from build123d import *

# Parameters (mm, degrees)
SKETCH1_R           = 1
BOSS_EXTRUDE1_DEPTH = 3
FILLET2_R           = 10


with BuildPart() as part:
    # Sketch1 → Boss-Extrude1 (new body)
    with BuildSketch(Plane.XY):
        with BuildLine():
            Line((0, 0), (5, 0))
            Line((5, 0), (5, -3))
            Line((5, -3), (20, -3))
            Line((20, -3), (20, 0))
            Line((20, 0), (25, 0))
            Line((25, 0), (25, 30))
            ThreePointArc((25, 30), (21.635660943, 33.364339057), (18.271321885, 30))
            Line((18.271321885, 30), (18.271321885, 25.388028695))
            Line((18.271321885, 25.388028695), (17.277972917, 24.007768839))
            ThreePointArc((17.277972917, 24.007768839), (2.760122096, 20.009620418), (3.579412381, 4.97359878))
            Line((3.579412381, 4.97359878), (0, 0))
        make_face()
        with Locations((12.5, 13)):
            Circle(SKETCH1_R, mode=Mode.SUBTRACT)
        with Locations((21.635660943, 30)):
            Circle(SKETCH1_R, mode=Mode.SUBTRACT)
    extrude(amount=BOSS_EXTRUDE1_DEPTH)

    # Fillet2
    # the kernel refuses this fillet: 10 mm, written as the material it adds along each edge
    with BuildSketch(Plane(origin=(3.579412381, 4.97359878, 0), x_dir=(-0.5841350348464551, -0.8116564920364591, 0), z_dir=(0, 0, 1))) as fillet2_piece_1_section:
        with BuildLine():
            CenterArc((6.344003322, -9.997660671), FILLET2_R, 91.239343662, 53.979959966)
            Line((-1.869411105, -4.293291867), (-2.033679393, -4.179204491))
            ThreePointArc((-2.033679393, -4.179204491), (-0.906628796, -2.158871285), (-0.19542514, 0.042532512))
            Line((-0.19542514, 0.042532512), (0, 0.2))
            ThreePointArc((0, 0.2), (3.063856958, 0.2), (6.123388127, 0.199953213))
            Line((6.123388127, 0.199953213), (6.127713915, 0))
        make_face()
    fillet2_piece_1 = extrude(amount=3, mode=Mode.PRIVATE)
    fillet2_piece_1 = split(fillet2_piece_1, bisect_by=Plane(origin=(2.134897735, 0, 1.5), z_dir=(0, 1, 0)), keep=Keep.TOP, mode=Mode.PRIVATE)
    add(fillet2_piece_1)
    with BuildSketch(Plane(origin=(17.277972917, 24.007768839, 0), x_dir=(0.5841350348464545, 0.8116564920364596, 0), z_dir=(0, 0, 1))) as fillet2_piece_2:
        with BuildLine():
            CenterArc((7.496633226, 8.148949762), FILLET2_R, 209.104536821, 25.472441877)
            Line((-1.240703884, 3.284904099), (-1.415450626, 3.187623185))
            ThreePointArc((-1.415450626, 3.187623185), (-0.686649014, 1.617411734), (-0.19542514, -0.042532512))
            Line((-0.19542514, -0.042532512), (0, -0.2))
            ThreePointArc((0, -0.2), (0.850273404, -0.2), (1.584625079, -0.162978995))
            Line((1.584625079, -0.162978995), (1.700546807, 0))
        make_face()
    extrude(amount=3)


solid = part.part
Work out the finished part from the listing and answer in its coordinate system (mm). A direction names the side the tool comes from. Coordinates: 2 decimals unless noted, no trailing zeros. Loops run counter-clockwise (first coordinate to the right, second up) from the corner with the lowest first, then second, coordinate; pieces in that order, holes last. Notation, with made-up numbers: M 28,20.5 L 33,20.5 A17 ccw 33,25.5 Z; hole C 17,80 d10. An arc over 180 degrees is marked long. Answer in a Markdown table with one row per item. Add a question column.
1. The mould has two halves that part along X. Classify faces 1 (the cylindrical face through (16.074, 24.906, 1.479)), 2 (the cylindrical face through (21.71, 33.364, 1.479)), 3 (the flat face through (16, 14, 3)), 4 (the cylindrical face through (21.505, 30.991, 1.479)): pulls with the +X half, pulls with the -X half, needs draft (parallel to the pull), parting line crosses it, or undercut.
2. Find section B-B, the plane y = 13. Write down the section's boundary in (x, z).
3. Consider L1, parallel to Y at x = 12.5, z = 1.45; L2, parallel to X at y = 27.5, z = 0.4; L3, parallel to X at y = 6, z = 2.45. Determine where each line is inside the solid, lowest interval first.
4. Find section D-D, the plane y = 2. Write down the section's boundary in (x, z).
5. Find section A-A, the plane x = 12.5. Write down the section's boundary in (y, z).
6. Flat-ended cylindrical pins translate along their axes: P1, Ø3, axis at x = 21.64, y = 30, coming from the -Z side; P2, Ø1.5, axis at y = -1.5, z = 1.5, coming from the +X side; P3, Ø1, axis at x = 5.5, y = 24.5, coming from the -Z side; P4, Ø1.5, axis at x = 22.5, z = 1.5, coming from the -Y side. Find the tip coordinate at first contact, or state that the pin passes through.
7. A tool of negligible diameter and unlimited length cuts with its end or side. For faces 5 (the flat face through (20, -2, 1)), 6 (the flat face through (16, 14, 0)), 7 (the flat face through (18.271, 28, 1)), 8 (the flat face through (2, 0, 1)), from which of +Z, -Z, +X, -X, +Y, -Y can it reach the whole face along a straight path? Write none if from no direction.
8. Find section C-C, the plane z = 2.1. Write down the section's boundary in (x, y), then the cut area to 3 significant figures.
Reported:
| question | item | result |
|---|---|---|
| 1 | face 1 | undercut |
| 1 | face 2 | parting line crosses it |
| 1 | face 3 | needs draft |
| 1 | face 4 | undercut |
| 2 | outline | M 0.5,0 L 11.5,0 L 11.5,3 L 0.5,3 Z; M 13.5,0 L 25,0 L 25,3 L 13.5,3 Z |
| 3 | L1 | y = -3 to 12, 14 to 25 |
| 3 | L2 | x = 18.27 to 25 |
| 3 | L3 | x = 1.75 to 25 |
| 4 | outline | M 1.06,0 L 25,0 L 25,3 L 1.06,3 Z |
| 5 | outline | M -3,0 L 12,0 L 12,3 L -3,3 Z; M 14,0 L 25,0 L 25,3 L 14,3 Z |
| 6 | P1 | stops at z = 0 |
| 6 | P2 | stops at x = 20 |
| 6 | P3 | passes through |
| 6 | P4 | stops at y = 0 |
| 7 | face 5 | +Z, -Z, +X, -Y |
| 7 | face 6 | -Z, +X, -X, +Y, -Y |
| 7 | face 7 | +Z, -Z, -X, +Y |
| 7 | face 8 | +Z, -Z, -X, -Y |
| 8 | outline | M 0,0 L 5,0 L 5,-3 L 20,-3 L 20,0 L 25,0 L 25,30 A3.36 ccw 18.27,30 L 18.27,25.39 A10 cw 13.89,24.92 A12 ccw 1.19,9 A10 cw Z; hole C 12.5,13 d2; hole C 21.64,30 d2 |
| 8 | area | 663 mm^2 |
